Study the drawing (mm; zero at the part's minimum x, y, z) and answer. A direction names the side the tool comes from. Coordinates: 2 decimals unless noted, no trailing zeros. Loops run counter-clockwise (first coordinate to the right, second up) from the corner with the lowest first, then second, coordinate; pieces in that order, holes last.
Q1. Section A-A (z = 1.3) is taken. Give the vertices of the cut face in (x, y), then the cut area to 3 significant figures.
Q2. Section B-B (x = 5.5) is taken. Give the vertices of the cut face in (y, z), then the cut area to 3 significant figures.
Q3. Flat-ended cylindrical pins translate along their axes: P1, Ø1, axis at x = 10.5, z = 2, coming from the -Y side; P2, Ø2, axis at x = 12, z = 0.5, coming from the +Y side; P3, Ø1.5, axis at y = 1, z = 1.5, coming from the -X side. Find the tip coordinate at first contact, or state that the pin passes through.
Q4. Which of the six approach directions +Z, -Z, +X, -X, +Y, -Y give full straight-line access (tool end or side, diameter ignored) to the marked faces 1, 2, 3 and 4?
Q5. Straight lines are drawn through the part: line 1 (Y direction, x = 8, z = 0.9); line 2 (X direction, y = 3.5, z = 5); line 3 (Z direction, x = 8, y = 4.5). For each, find the intervals that lie inside material, in ascending order.
Q6. Section D-D (z = 2.4) is taken. Give the vertices of the cut face in (x, y), then the cut area to 3 significant figures.
Q7. Section C-C (y = 3.5) is taken. Give the vertices of the cut face in (x, z).
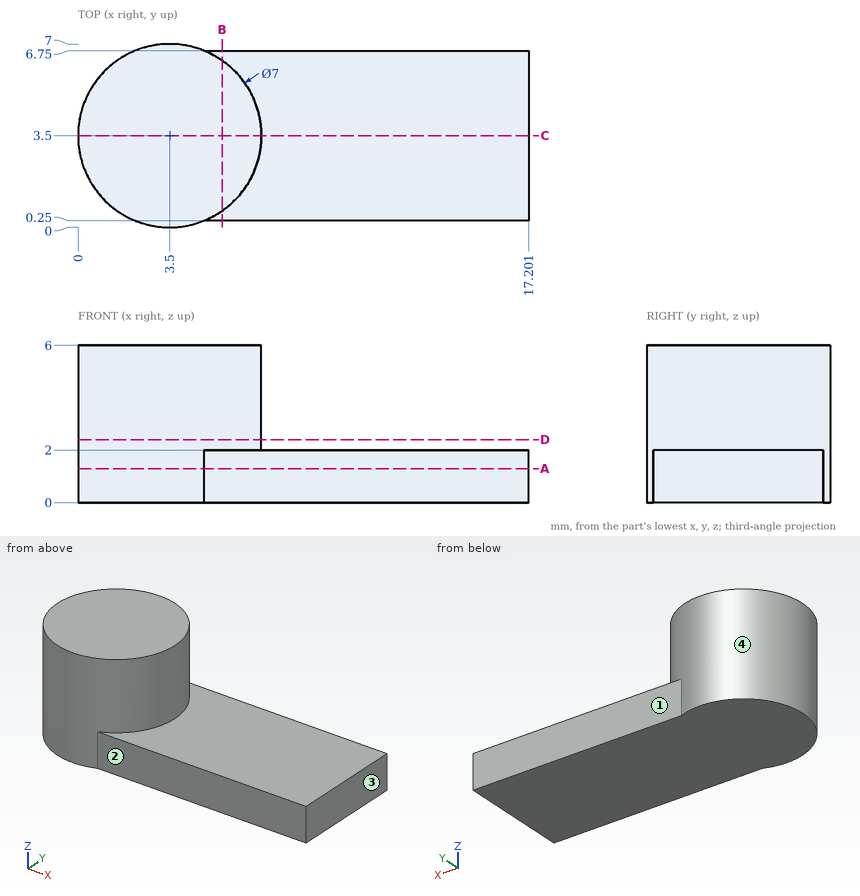
Numbers:
1. outline: (4.8, 0.25) - (17.2, 0.25) - (17.2, 6.75) - (4.8, 6.75) arc R3.5 ccw (long way) to start
1. area: 109 mm2
2. outline: (0.25, 0) - (6.75, 0) - (6.75, 2) - (6.37, 2) - (6.37, 6) - (0.63, 6) - (0.63, 2) - (0.25, 2) - close
2. area: 36.0 mm2
3. P1: stops at y = 0.25
3. P2: stops at y = 6.75
3. P3: stops at x = 0.47
4. face 1: +Z, -Z, +X, +Y
4. face 2: +Z, -Z, +X, -Y
4. face 3: +Z, -Z, +X, +Y, -Y
4. face 4: +Z
5. line 1: y = 0.25 to 6.75
5. line 2: x = 0 to 7
5. line 3: z = 0 to 2
6. outline: circle Ø7 at (3.5, 3.5)
6. area: 38.5 mm2
7. outline: (0, 0) - (17.2, 0) - (17.2, 2) - (7, 2) - (7, 6) - (0, 6) - close
